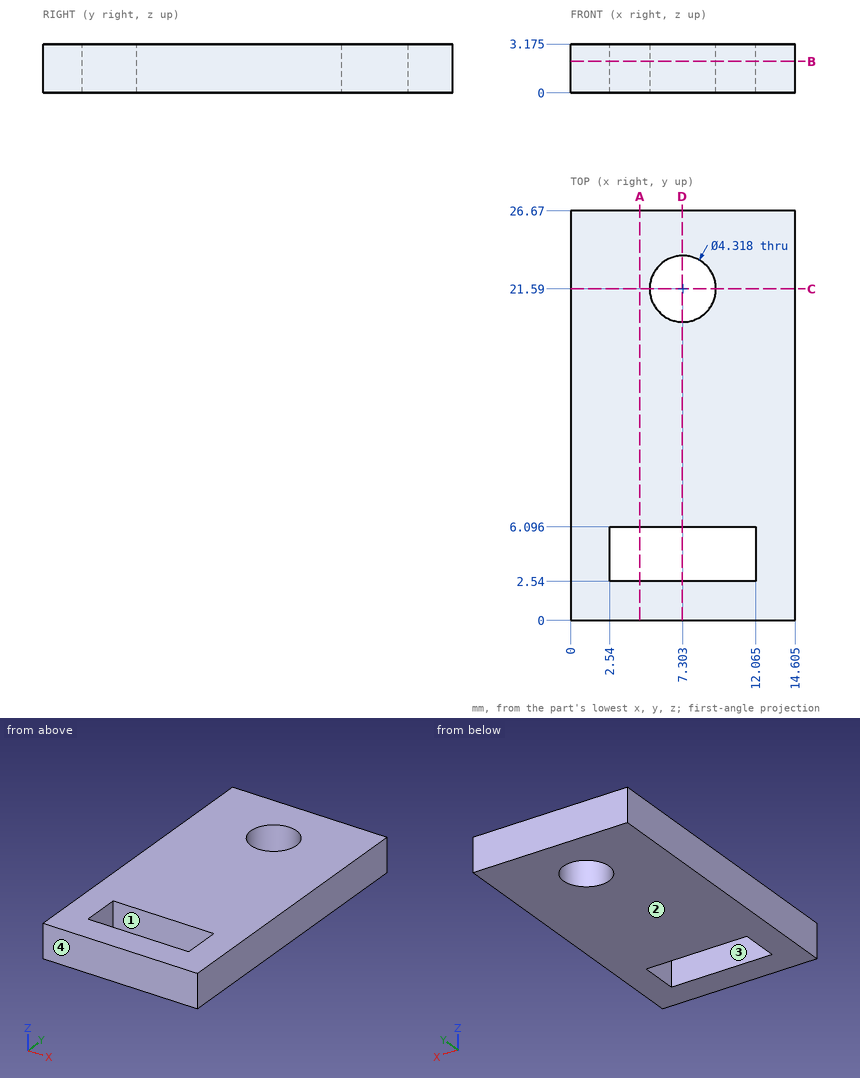
Part print with two shaded views. Sizes in mm from the minimum x, y, z corner. Coordinates: 2 decimals unless noted, no trailing zeros. Write each loop counter-clockwise with the first axis right and the second up, starting at its lowest first coordinate (ties: lowest second). Pieces come first, ordered by that corner, then holes. Notation, with made-up numbers: (81.25, 11) -> (123.25, 11) arc R27 cw to (123.25, 42) -> close; hole circle Ø7 at (-24, 74). An arc over 180 degrees is marked (long way). Return JSON: item names as keys, results as strings. Group by question number.
Q1. Pull direction Y, two halves, no side cores. Call the marked faces 1, 2, 3 and 4: released by +Y, released by -Y, zero draft, split by the parting line, or undercut.
Q2. Cut at C-C, the plane y = 21.59. Give the cut face in (x, z) (1 decimal).
Q3. Flat gauge pin, fed straight in: pin 1 (3.5 mm diameter, centred on x = 7.3, y = 21.59, fed in from -Z). Where does the tip first touch, or does it go through?
Q4. Cut at D-D, the plane x = 7.25. Give the cut face in (y, z) (1 decimal).
Q5. Cut at B-B, the plane z = 2.05. Give the cut face in (x, y) (1 decimal).
Q6. Cut at A-A, the plane x = 4.5. Give the cut face in (y, z) (1 decimal).
Q7. Drill centre lines: line 1 (Y direction, x = 5.5, z = 0.45) (1 decimal); line 2 (Y direction, x = 4, z = 2.4) (1 decimal); line 3 (Y direction, x = 9, z = 0.9) (1 decimal). Where is each one in solid material? Low to high.
Returned:
{
 "1": {"face 1": "undercut", "face 2": "zero draft", "face 3": "undercut", "face 4": "released by -Y"},
 "2": {"outline": "(0, 0) -> (5.1, 0) -> (5.1, 3.2) -> (0, 3.2) -> close; (9.5, 0) -> (14.6, 0) -> (14.6, 3.2) -> (9.5, 3.2) -> close"},
 "3": {"pin 1": "passes through"},
 "4": {"outline": "(0, 0) -> (2.5, 0) -> (2.5, 3.2) -> (0, 3.2) -> close; (6.1, 0) -> (19.4, 0) -> (19.4, 3.2) -> (6.1, 3.2) -> close; (23.7, 0) -> (26.7, 0) -> (26.7, 3.2) -> (23.7, 3.2) -> close"},
 "5": {"outline": "(0, 0) -> (14.6, 0) -> (14.6, 26.7) -> (0, 26.7) -> close; hole (2.5, 2.5) -> (12.1, 2.5) -> (12.1, 6.1) -> (2.5, 6.1) -> close; hole circle Ø4.3 at (7.3, 21.6)"},
 "6": {"outline": "(0, 0) -> (2.5, 0) -> (2.5, 3.2) -> (0, 3.2) -> close; (6.1, 0) -> (26.7, 0) -> (26.7, 3.2) -> (6.1, 3.2) -> close"},
 "7": {"line 1": "y = 0 to 2.5, 6.1 to 20.4, 22.8 to 26.7", "line 2": "y = 0 to 2.5, 6.1 to 26.7", "line 3": "y = 0 to 2.5, 6.1 to 20.3, 22.9 to 26.7"}
}
